Build history of the part. All positions in model axes, mm. Round coordinates to 2 decimals unless told otherwise and drop trailing zeros. Write each loop counter-clockwise with the first axis right and the second up, starting at its lowest first coordinate (ties: lowest second). Pieces come first, ordered by that corner, then holes. Notation, with made-up numbers: (-19, 74) - (40, 74) arc R18 cw to (40, 92) - close; hole circle Ø1 at (4, 72). An arc over 180 degrees is marked (long way). One line per question, with ' | ' between items.
Autodesk Inventor part; units mm, degrees
ref_plane "YZ Plane" through (0, 0, 0) normal (1, 0, 0) x (0, 1, 0)
ref_plane "XZ Plane" through (0, 0, 0) normal (0, 1, 0) x (-1, 0, 0)
ref_plane "XY Plane" through (0, 0, 0) normal (0, 0, 1) x (1, 0, 0)
sketch "Sketch1" plane through (0, 0, 0) normal (0, 1, 0) x (-1, 0, 0)
  circle A0 centre (0.1602, 0) radius 3
  point P0 (0, 0)
  dimension "d0" = 6
extrude "Extrusion2" add sketch "Sketch1" along normal blind 16.6
fillet "Fillet1" radius 0.5 1 edges at (2.8398, 16.6, 0)
fillet "Fillet2" radius 0.5 1 edges at (2.8398, 0, 0)
properties part number "connector"
Q1. Drill centre lines: L1, parallel to X at y = 15.5, z = -0.8; L2, parallel to Z at x = -1.1, y = 15; L3, parallel to Y at x = 1.65, z = 2.3. Where is each one in solid material? Low to high. Write a range as from..to.
Found:
L1: -3.05..2.73 | L2: -2.85..2.85 | L3: 0.24..16.36
Q2. Saw through at A-A, the plane y = 7.25. List the corners of the cut face in (x, z), then the cut area to 3 significant figures.
Found:
outline: circle Ø6 at (-0.16, 0) | area: 28.3 mm^2
Q3. Drop flat-ended pins along their axis: pin 1 (2 mm diameter, centred on y = 11, z = -1.5, fed in from +X); pin 2 (1.5 mm diameter, centred on y = 9.5, z = -1.5, fed in from +X). Give the stop position or say it passes through.
Found:
pin 1: x = 2.8 | pin 2: x = 2.74
